Design review of the part built by this model. Coordinates are the model's own, in mm. Coordinates: 2 decimals unless noted, no trailing zeros. Order: outer loops, then holes, each group sorted by start corner. A loop starts at its lowest first (then second) coordinate and runs counter-clockwise, first axis right, second up. Notation, with made-up numbers: (-14, 75.25) -> (5, 75.25) arc R21 ccw to (5, 105.25) -> close; hole circle Ø11 at (-31, 31.25). An arc over 180 degrees is marked (long way). Use a Markdown table: item, result. Add a question column.
Q1. Add section D-D (x = -27). State the section outline as (y, z) points, then the cut area to 3 significant figures.
Q2. Insertion check: pin 1 (10 mm diameter, centred on x = -175.5, z = 46.5, fed in from -Y); pin 2 (3 mm diameter, centred on x = -55.5, z = 57, fed in from -Y); pin 3 (3 mm diameter, centred on x = -12, y = 7.5, fed in from -Z). Each pin has a flat end and moves straight along its axis. Give the tip position at first contact, or say it passes through.
Q3. Add section B-B (y = -3.5). State the section outline as (x, z) points, then the cut area to 3 significant figures.
Q4. Wall thickness on probe 1 along Y at (x, z) = (-96, 40.5); probe 2 along X at (y, z) = (-3.5, 61.3): over which ranges is each line inside the solid? List them lowest first.
Q5. Add section C-C (z = 50). Count the separate pieces of the cut face and the enclosed holes in it, then the cut area to 3 significant figures.
Q6. Add section A-A (x = -4). State the section outline as (y, z) points, then the cut area to 3 significant figures.
from build123d import *

# Parameters (mm, degrees)
BOSS_EXTRUDE1_DEPTH = 4
BOSS_EXTRUDE2_START = -45
BOSS_EXTRUDE2_DEPTH = 3
BOSS_EXTRUDE3_START = -39
BOSS_EXTRUDE3_DEPTH = 3
BOSS_EXTRUDE4_REACH = 212.155
SKETCH6_R           = 2.5
SKETCH7_W           = 10
SKETCH7_H           = 4
CUT_EXTRUDE1_DEPTH  = 10
SKETCH8_R           = 7.5


with BuildPart() as part:
    # Sketch1 → Boss-Extrude1 (new body)
    with BuildSketch(Plane(origin=(0, 0, 0), x_dir=(1, 0, 0), z_dir=(0, 1, 0))):
        with BuildLine():
            Line((-110, 0), (0, 0))
            Line((0, 0), (0, -105))
            Line((0, -105), (-110, -105))
            add(Edge.make_bspline(
                [(-190, -72.5), (-172.262756658, -100.700379519), (-139.265999107, -104.836107107), (-110, -105)],
                knots=[0, 0, 0, 0, 1, 1, 1, 1], degree=3))
            Line((-190, -72.5), (-190, -32.5))
            add(Edge.make_bspline(
                [(-190, -32.5), (-171.707374586, -4.618888995), (-138.989901699, -2.178666842), (-110, 0)],
                knots=[0, 0, 0, 0, 1, 1, 1, 1], degree=3))
        make_face()
    extrude(amount=BOSS_EXTRUDE1_DEPTH)

    # Sketch2 → Boss-Extrude2 (add, symmetric)
    with BuildSketch(Plane.XY.offset(105).offset(BOSS_EXTRUDE2_START)):
        with BuildLine():
            Line((-190, 4), (-200, 4))
            Line((-200, 4), (-200, 1))
            ThreePointArc((-200, 1), (-194.2, -3.5), (-200, -8))
            Line((-200, -8), (-200, -11))
            Line((-200, -11), (-190, -11))
            Line((-190, -11), (-178, 0))
            Line((-178, 0), (-190, 4))
        make_face()
    boss_extrude2 = extrude(amount=BOSS_EXTRUDE2_DEPTH, both=True)

    # Mirror1: Boss-Extrude2 across plane
    add(boss_extrude2.mirror(Plane.XY.offset(52.5)))

    # Sketch5 → Boss-Extrude3 (add, symmetric)
    with BuildSketch(Plane.XY.offset(105).offset(BOSS_EXTRUDE3_START)):
        Polygon((-16.979807258, 4), (-7.979807258, 14), (0, 14), (0, 4), align=None)
    boss_extrude3 = extrude(amount=BOSS_EXTRUDE3_DEPTH, both=True)

    # Mirror4: Boss-Extrude3 across plane
    add(boss_extrude3.mirror(Plane.XY.offset(52.5)))

    # Sketch6 → Boss-Extrude4 (add, up to next)
    with BuildSketch(Plane.XY.offset(42), mode=Mode.PRIVATE) as boss_extrude4_sk1:
        with Locations(Location((-4, 10, 0), (0, 0, 180))):
            Circle(SKETCH6_R)
    boss_extrude4_tool1 = extrude(boss_extrude4_sk1.sketch, amount=BOSS_EXTRUDE4_REACH, mode=Mode.PRIVATE) - part.part
    add(boss_extrude4_tool1.solids().sort_by_distance((-4, 10, 42))[0])

    # Sketch7 → Cut-Extrude1 (cut)
    with BuildSketch(Plane(origin=(0, 4, 0), x_dir=(1, 0, 0), z_dir=(0, 1, 0))):
        with Locations((-99, -99)):
            Rectangle(SKETCH7_W, SKETCH7_H)
    cut_extrude1 = extrude(amount=-CUT_EXTRUDE1_DEPTH, mode=Mode.SUBTRACT)

    # Mirror5: Cut-Extrude1 across plane
    add(cut_extrude1.mirror(Plane.XY.offset(52.5)), mode=Mode.SUBTRACT)

    # Cut-Sweep1: sweep along a path in Sketch9
    with BuildLine(Plane.XY.offset(52.5)) as cut_sweep1_path:
        Line((-150, 4), (-163.867437875, -3.466183031))
    # Sketch8 → Cut-Sweep1 (sweep, cut)
    with BuildSketch(Plane(origin=(0, 4, 0), x_dir=(1, 0, 0), z_dir=(0, 1, 0))):
        with Locations((-150, -52.5)):
            Circle(SKETCH8_R)
    sweep(path=cut_sweep1_path.line, mode=Mode.SUBTRACT)


solid = part.part
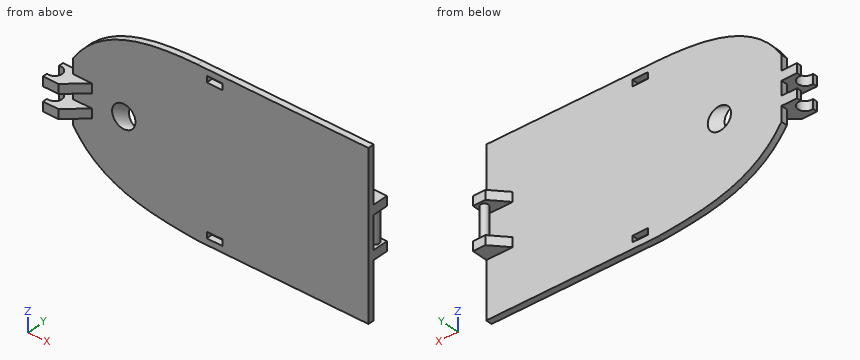
Established:
| question | item | result |
|---|---|---|
| 1 | outline | (0, 0) -> (4, 0) -> (4, 105) -> (0, 105) -> close |
| 1 | area | 420 mm^2 |
| 2 | pin 1 | y = -2.29 |
| 2 | pin 2 | y = 0 |
| 2 | pin 3 | z = 36 |
| 3 | outline | (-194.2, 42) -> (-181.82, 42) -> (-181.82, 48) -> (-194.2, 48) -> close; (-194.2, 57) -> (-181.82, 57) -> (-181.82, 63) -> (-194.2, 63) -> close |
| 3 | area | 149 mm^2 |
| 4 | probe 1 | 0 to 4 |
| 4 | probe 2 | -194.2 to -181.82 |
| 5 | separate pieces | 3 |
| 5 | enclosed holes | 0 |
| 5 | area | 723 mm^2 |
| 6 | outline | (0, 0) -> (4, 0) -> (4, 36) -> (14, 36) -> (14, 42) -> (12.5, 42) -> (12.5, 63) -> (14, 63) -> (14, 69) -> (4, 69) -> (4, 105) -> (0, 105) -> close; hole (4, 42) -> (7.5, 42) -> (7.5, 63) -> (4, 63) -> close |
| 6 | area | 645 mm^2 |
